from build123d import *

# Parameters (mm, degrees)
F0_W     = 254
F0_H     = 762
F1_DEPTH = 1016
F2_R     = 254
F3_DEPTH = 1064.26
F5_DEPTH = 508
F7_DEPTH = 254
F9_DEPTH = 762


with BuildPart() as f1:
    # F0 (on Front) → F1 (new body)
    with BuildSketch(Plane.XZ):
        with BuildLine():
            Line((0, 1016), (0, 254))
            Line((0, 254), (1016, 254))
            Line((1016, 254), (1016, 1016))
            Line((1016, 1016), (762, 1016))
            ThreePointArc((762, 1016), (508, 762), (254, 1016))
            Line((254, 1016), (0, 1016))
        make_face()
        Polygon((0, 254), (0, 0), (1778, 0), (1778, 254), (1270, 254), (1016, 254), align=None)
        with Locations((1143, 635)):
            Rectangle(F0_W, F0_H)
        Polygon((1270, 254), (1778, 254), (1270, 1016), align=None)
    extrude(amount=F1_DEPTH)

    # F2 (on face) → F3 (cut)
    with BuildSketch(Plane.XZ.offset(1016)):
        with Locations((508, 1016)):
            Circle(F2_R)
    extrude(amount=-F3_DEPTH, mode=Mode.SUBTRACT)

    # F4 (on face) → F5 (cut)
    with BuildSketch(Plane.XZ.offset(1016)):
        Polygon((1270, 254), (1270, 1016), (254, 1016), (0, 1016), (0, 254), align=None)
        Polygon((1778, 254), (1270, 1016), (1270, 254), align=None)
    extrude(amount=-F5_DEPTH, mode=Mode.SUBTRACT)

    # F6 (on face) → F7 (cut)
    with BuildSketch(Plane.XZ.offset(508)):
        Polygon((1778, 254), (1270, 1016), (1270, 254), align=None)
    extrude(amount=-F7_DEPTH, mode=Mode.SUBTRACT)

    # F8 (on face) → F9 (cut)
    with BuildSketch(Plane.XY.offset(1016)):
        Polygon((1270, -508), (1270, -254), (1016, -508), align=None)
    extrude(amount=-F9_DEPTH, mode=Mode.SUBTRACT)


solid = f1.part
Input: part model. Units: mm. Frame: model coordinates. A direction names the side the tool comes from. Coordinates: 2 decimals unless noted, no trailing zeros. Order: outer loops, then holes, each group sorted by start corner. A loop starts at its lowest first (then second) coordinate and runs counter-clockwise, first axis right, second up. Notation, with made-up numbers: M 77.25,6.5 L 103.25,6.5 A28 cw 103.25,44.5 Z; hole C -12.5,45.5 d9. An arc over 180 degrees is marked long. Answer as CSV lines item,"result".
1. Access query for faces 1 (the flat face through (877, -501, 0)), 2 (the flat face through (1145, -379, 640)). Directions: +Z, -Z, +X, -X, +Y, -Y. A direction counts if a zero-diameter tool reaches every point of the face in a straight line with its end or side. Return the directions, or none.
Reported:
face 1,"-Z, +X, -X, +Y, -Y"
face 2,"+Z, +X, -Y"
2. Section B-B (x = 1510). Return the cut outline in (y, z), then the cut area to 3 significant figures.
Reported:
outline,"M -1016,0 L 0,0 L 0,656 L -254,656 L -254,254 L -1016,254 Z"
area,"360,000 mm2"
3. Pull-direction query (X, two-part tool) for faces 3 (the cylindrical face through (513.59, -250.44, 762.06)), 4 (the flat face through (501, -508, 556)), 5 (the flat face through (1778, -501, 125)); classes: released by +X, released by -X, zero draft, split by the parting line, or undercut.
Reported:
face 3,"undercut"
face 4,"zero draft"
face 5,"released by +X"
4. Section A-A (y = -418). Return the cut outline in (x, z), then the cut area to 3 significant figures.
Reported:
outline,"M 0,0 L 1778,0 L 1778,254 L 1106,254 L 1106,1016 L 762,1016 A254 cw 254,1016 L 0,1016 Z"
area,"1,190,000 mm2"
5. Section C-C (z = 416.5). Return the cut outline in (x, y), then the cut area to 3 significant figures.
Reported:
outline,"M 0,-508 L 1016,-508 L 1270,-254 L 1669.67,-254 L 1669.67,0 L 0,0 Z"
area,"714,000 mm2"
6. First-contact query: P1, Ø1.5, axis at x = 1135, z = 264, coming from the -Y side; P2, Ø6, axis at x = 1087.5, y = -816.5, coming from the +Z side; P3, Ø6, axis at x = 1060.5, y = -910, coming from the -Z side; P4, Ø5, axis at x = 877, z = 357, coming from the -Y side. Flat tips, straight axial feed; report the tip coordinate or a pass-through.
Reported:
P1,"y = -389.75"
P2,"z = 254"
P3,"z = 0"
P4,"y = -508"
7. Section D-D (y = -883). Return the cut outline in (x, z), then the cut area to 3 significant figures.
Reported:
outline,"M 0,0 L 1778,0 L 1778,254 L 0,254 Z"
area,"452,000 mm2"
8. Material intervals for line 1 (Y direction, x = 1403, z = 519); line 2 (Y direction, x = 590, z = 753.5); line 3 (X direction, y = -443.5, z = 913), sorted ascending. Write a range as from..to.
Reported:
line 1,"-254..0"
line 2,"-508..0"
line 3,"0..275.82, 740.18..1080.5"
